The model under review builds one solid part; all positions refer to its coordinate system, in mm. Face numbers are marked on the shaded views. A direction names the side the tool comes from. Coordinates: 2 decimals unless noted, no trailing zeros. Loops run counter-clockwise (first coordinate to the right, second up) from the corner with the lowest first, then second, coordinate; pieces in that order, holes last. Notation, with made-up numbers: (63.25, -21.5) - (81.25, -21.5) arc R23 ccw to (81.25, -2.5) - close; hole circle Ø4 at (27, 60.5). An arc over 180 degrees is marked (long way). One line per item, written item: value. Start each with the question number.
1. For the marked faces 5, 6, 7, 8 and 9, list the 3-axis set-ups (+Z, -Z, +X, -X, +Y, -Y) from which the entire face can be reached by the end or side of a thin tool; tool diameter is ignored.
2. Insertion check: P1, Ø0.9, axis at y = -6, z = 1, coming from the +X side; P2, Ø11.5, axis at x = 2.5, y = -8.5, coming from the +Z side; P3, Ø3, axis at x = -1.5, z = 24.5, coming from the +Y side; P4, Ø1.5, axis at x = -7.5, z = 19.5, coming from the +Y side. Each pin has a flat end and moves straight along its axis. Give the tip position at first contact, or say it passes through.
3. We need section C-C, the plane z = 22.25. Give the boundary of the cut face in (x, y), then the cut area to 3 significant figures.
4. To check wall thickness, follow line 1 (X direction, y = -23.5, z = 23.25); line 2 (Y direction, x = 4.5, z = 25); line 3 (Z direction, x = 2, y = -18.25). State the ranges of each line that lie inside material, in increasing order.
5. Mouldability with a two-part tool opening along Z and no side actions: class the marked faces 1, 2, 3 and 4 as +Z half, -Z half, draft (parallel to the pull), parting line (faces both ways), or undercut.
6. We need section B-B, the plane y = -22.75. Give the boundary of the cut face in (x, z).
7. We need section D-D, the plane y = -10. Give the boundary of the cut face in (x, z).
8. We need section A-A, the plane x = 0. Give the boundary of the cut face in (y, z).
from build123d import *

# Parameters (mm, degrees)
EXTRUDE_1_DEPTH     = 3
SKETCH_1_3_W        = 12.007345154
SKETCH_1_3_H        = 3
EXTRUDE_2_DEPTH     = 30
SKETCH_2_R          = 1.75
CUT_EXTRUDE_1_DEPTH = 15
FILLET_1_R          = 5
CHAMFER_1_SIZE      = 2


with BuildPart() as part:
    # Sketch 1 → Extrude 1 (new body)
    with BuildSketch(Plane.XY):
        with BuildLine():
            ThreePointArc((4, 0), (0, 4), (-4, 0))
            Line((-4, 0), (-12.007345154, -22))
            Line((-12.007345154, -22), (12.007345154, -22))
            Line((12.007345154, -22), (4, 0))
        make_face()
        with BuildLine():
            Line((-1.75, -15), (-1.75, 0))
            ThreePointArc((-1.75, 0), (0, 1.75), (1.75, 0))
            Line((1.75, 0), (1.75, -15))
            ThreePointArc((1.75, -15), (0, -16.75), (-1.75, -15))
        make_face(mode=Mode.SUBTRACT)
    extrude(amount=EXTRUDE_1_DEPTH)

    # Sketch 1_3 → Extrude 2 (add)
    with BuildSketch(Plane.XY):
        with Locations((-6.003672577, -23.5)):
            Rectangle(SKETCH_1_3_W, SKETCH_1_3_H)
        with Locations((6.003672577, -23.5)):
            Rectangle(SKETCH_1_3_W, SKETCH_1_3_H)
    extrude(amount=EXTRUDE_2_DEPTH)

    # Sketch 2 → Cut-Extrude 1 (cut)
    with BuildSketch(Plane(origin=(0, -22, 0), x_dir=(1, 0, 0), z_dir=(0, 1, 0))):
        with Locations((-7.007345154, -7)):
            Circle(SKETCH_2_R)
        with BuildLine():
            Line((-5.257345154, -26), (-5.257345154, -7))
            ThreePointArc((-5.257345154, -7), (-7.007345154, -8.75), (-8.757345154, -7))
            Line((-8.757345154, -7), (-8.757345154, -26))
            ThreePointArc((-8.757345154, -26), (-7.007345154, -24.25), (-5.257345154, -26))
        make_face()
        with Locations((-7.007345154, -26)):
            Circle(SKETCH_2_R)
        with Locations((7.007345154, -26)):
            Circle(SKETCH_2_R)
        with BuildLine():
            ThreePointArc((8.757345154, -7), (7.007345154, -8.75), (5.257345154, -7))
            Line((5.257345154, -7), (5.257345154, -26))
            ThreePointArc((5.257345154, -26), (7.007345154, -24.25), (8.757345154, -26))
            Line((8.757345154, -26), (8.757345154, -7))
        make_face()
        with Locations((7.007345154, -7)):
            Circle(SKETCH_2_R)
    extrude(amount=-CUT_EXTRUDE_1_DEPTH, mode=Mode.SUBTRACT)

    # Fillet 1
    fillet_1_edges = [part.edges().sort_by_distance(p)[0] for p in [
        (12.007345154, -23.5, 30),
        (-12.007345154, -23.5, 30),
    ]]
    fillet(fillet_1_edges, radius=FILLET_1_R)

    # Chamfer 1
    chamfer_1_edges = [part.edges().sort_by_distance(p)[0] for p in [
        (0, -22, 3),
    ]]
    chamfer(chamfer_1_edges, length=CHAMFER_1_SIZE)


solid = part.part
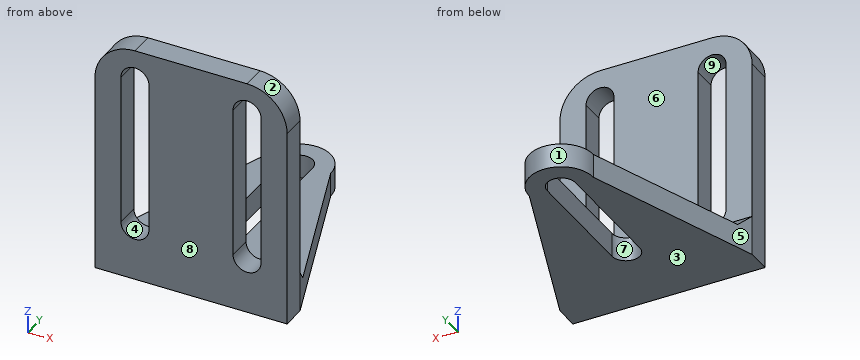
Findings below:
1. face 5: +Z, -Z, -X, +Y
1. face 6: +Z, +X, -X, +Y
1. face 7: +Z, -Z
1. face 8: +Z, -Z, +X, -X, -Y
1. face 9: +Y, -Y
2. P1: x = 6.35
2. P2: z = 3
2. P3: y = -22
2. P4: through
3. outline: (-12.01, -25) - (-8.76, -25) - (-8.76, -22) - (-12.01, -22) - close; (-5.26, -25) - (5.26, -25) - (5.26, -22) - (-5.26, -22) - close; (8.76, -25) - (12.01, -25) - (12.01, -22) - (8.76, -22) - close
3. area: 51.0 mm2
4. line 1: -12.01 to -8.76, -5.26 to 5.26, 8.76 to 12.01
4. line 2: -25 to -22
4. line 3: 0 to 3
5. face 1: draft
5. face 2: +Z half
5. face 3: -Z half
5. face 4: undercut
6. outline: (-12.01, 0) - (12.01, 0) - (12.01, 25) arc R5 ccw to (7.01, 30) - (-7.01, 30) arc R5 ccw to (-12.01, 25) - close; hole (-8.76, 7) arc R1.75 ccw to (-5.26, 7) - (-5.26, 26) arc R1.75 ccw to (-8.76, 26) - close; hole (5.26, 7) arc R1.75 ccw to (8.76, 7) - (8.76, 26) arc R1.75 ccw to (5.26, 26) - close
7. outline: (-7.64, 0) - (-1.75, 0) - (-1.75, 3) - (-7.64, 3) - close; (1.75, 0) - (7.64, 0) - (7.64, 3) - (1.75, 3) - close
8. outline: (-25, 0) - (-16.75, 0) - (-16.75, 3) - (-20, 3) - (-22, 5) - (-22, 30) - (-25, 30) - close; (1.75, 0) - (4, 0) - (4, 3) - (1.75, 3) - close
